For this review, take the finished solid that the model builds, in its own axes (mm). A direction names the side the tool comes from. Coordinates: 2 decimals unless noted, no trailing zeros. Loops run counter-clockwise (first coordinate to the right, second up) from the corner with the lowest first, then second, coordinate; pieces in that order, holes last. Notation, with made-up numbers: M -15.5,-3.5 L 15.5,-3.5 A19 ccw 15.5,30.5 Z; hole C -17.75,89.5 d11. An arc over 180 degrees is marked long. Put each result on its own line as item: value.
```python
from build123d import *

# Parameters (mm, degrees)
SKETCH1_R                                         = 5.08
SKETCH1_R_2                                       = 1.524
BOSS_EXTRUDE1_DEPTH                               = 1.4732
CSK_FOR_4_FLAT_HEAD_MACHINE_SCREW_100_D           = 3.4544
CSK_FOR_4_FLAT_HEAD_MACHINE_SCREW_100_DEPTH       = 3.44932
CSK_FOR_4_FLAT_HEAD_MACHINE_SCREW_100_CSINK_D     = 5.715
CSK_FOR_4_FLAT_HEAD_MACHINE_SCREW_100_CSINK_ANGLE = 100
CSK_FOR_4_FLAT_HEAD_MACHINE_SCREW_100_TIP         = 1.037806461


with BuildPart() as part:
    # Sketch1 → Boss-Extrude1 (new body)
    with BuildSketch(Plane(origin=(0, 0, 0), x_dir=(1, 0, 0), z_dir=(0, 1, 0))):
        with BuildLine():
            Line((-3.81, 7.493), (-3.81, 16.383))
            ThreePointArc((-3.81, 16.383), (-2.731274275, 18.987274275), (-0.127, 20.066))
            Line((-0.127, 20.066), (0.127, 20.066))
            ThreePointArc((0.127, 20.066), (2.731274275, 18.987274275), (3.81, 16.383))
            Line((3.81, 16.383), (3.81, 7.493))
            ThreePointArc((3.81, 7.493), (4.888725725, 4.888725725), (7.493, 3.81))
            Line((7.493, 3.81), (16.383, 3.81))
            ThreePointArc((16.383, 3.81), (18.987274275, 2.731274275), (20.066, 0.127))
            Line((20.066, 0.127), (20.066, -0.127))
            ThreePointArc((20.066, -0.127), (18.987274275, -2.731274275), (16.383, -3.81))
            Line((16.383, -3.81), (7.493, -3.81))
            ThreePointArc((7.493, -3.81), (4.888725725, -4.888725725), (3.81, -7.493))
            Line((3.81, -7.493), (3.81, -16.383))
            ThreePointArc((3.81, -16.383), (2.731274275, -18.987274275), (0.127, -20.066))
            Line((0.127, -20.066), (-0.127, -20.066))
            ThreePointArc((-0.127, -20.066), (-2.731274275, -18.987274275), (-3.81, -16.383))
            Line((-3.81, -16.383), (-3.81, -7.493))
            ThreePointArc((-3.81, -7.493), (-4.888725725, -4.888725725), (-7.493, -3.81))
            Line((-7.493, -3.81), (-16.383, -3.81))
            ThreePointArc((-16.383, -3.81), (-18.987274275, -2.731274275), (-20.066, -0.127))
            Line((-20.066, -0.127), (-20.066, 0.127))
            ThreePointArc((-20.066, 0.127), (-18.987274275, 2.731274275), (-16.383, 3.81))
            Line((-16.383, 3.81), (-7.493, 3.81))
            ThreePointArc((-7.493, 3.81), (-4.888725725, 4.888725725), (-3.81, 7.493))
        make_face()
        Circle(SKETCH1_R, mode=Mode.SUBTRACT)
        with Locations((0, 17.0815)):
            Circle(SKETCH1_R_2, mode=Mode.SUBTRACT)
        with Locations((17.0815, 0)):
            Circle(SKETCH1_R_2, mode=Mode.SUBTRACT)
        with Locations((-17.0815, 0)):
            Circle(SKETCH1_R_2, mode=Mode.SUBTRACT)
        with Locations((0, -17.0815)):
            Circle(SKETCH1_R_2, mode=Mode.SUBTRACT)
    extrude(amount=BOSS_EXTRUDE1_DEPTH)

    # CSK for #4 Flat Head Machine Screw (100)2
    with Locations(Plane(origin=(0, 1.4732, 0), x_dir=(1, 0, 0), z_dir=(0, 1, 0))):
        with Locations((0, 8.001), (0, -8.001), (9.271, 0), (-9.271, 0)):
            CounterSinkHole(CSK_FOR_4_FLAT_HEAD_MACHINE_SCREW_100_D / 2, CSK_FOR_4_FLAT_HEAD_MACHINE_SCREW_100_CSINK_D / 2, depth=CSK_FOR_4_FLAT_HEAD_MACHINE_SCREW_100_DEPTH, counter_sink_angle=CSK_FOR_4_FLAT_HEAD_MACHINE_SCREW_100_CSINK_ANGLE)
            with Locations((0, 0, -(CSK_FOR_4_FLAT_HEAD_MACHINE_SCREW_100_DEPTH + CSK_FOR_4_FLAT_HEAD_MACHINE_SCREW_100_TIP / 2))):  # 118° drill point
                Cone(0, CSK_FOR_4_FLAT_HEAD_MACHINE_SCREW_100_D / 2, CSK_FOR_4_FLAT_HEAD_MACHINE_SCREW_100_TIP, mode=Mode.SUBTRACT)


solid = part.part
```
(1) Wall thickness on line 1 along Z through (x, y) = (0, 0.15); line 2 along Z through (x, y) = (-1, 0.5); line 3 along X through (y, z) = (0.45, -8): over which ranges is each line inside the solid? List them lowest first. Write a range as [from, to].
Determined:
line 1: z = [-20.07, -18.61], [-15.56, -9.73], [-6.27, -5.08], [5.08, 6.27], [9.73, 15.56], [18.61, 20.07]
line 2: z = [-19.96, -18.23], [-15.93, -9.41], [-6.59, -4.98], [4.98, 6.59], [9.41, 15.93], [18.23, 19.96]
line 3: x = [-3.81, -1.73], [1.73, 3.81]
(2) Tool access review of faces 5 (the flat face through (2, 0, -6)), 6 (the flat face through (-3.81, 1, -12)): name each direction out of +Z, -Z, +X, -X, +Y, -Y from which nothing blocks a thin tool from reaching the whole face with its end or side.
Determined:
face 5: +Z, -Z, +X, -X, -Y
face 6: -Z, -X, +Y, -Y
(3) Draft analysis for pull direction Z (two halves, no side actions). For faces 1 (the flat face through (3.81, 1, -12)), 2 (the cylindrical face through (-0.198, 0.726, -18.593)), 3 (the cylindrical face through (19.02, 0.73, 2.7)), 4 (the cylindrical face through (0.37, 0.26, 9.69)), state which applies: +Z half, -Z half, draft (parallel to the pull), parting line (faces both ways), or undercut.
Determined:
face 1: draft
face 2: undercut
face 3: +Z half
face 4: undercut
(4) Add section C-C (z = 12). Write out the cut boundary in (x, y), plus the area to 3 significant figures.
Determined:
outline: M -3.81,0 L 3.81,0 L 3.81,1.47 L -3.81,1.47 Z
area: 11.2 mm^2
(5) Add section A-A (y = 0.25). State how many separate pieces and enclosed holes the cut face has, plus the area to 3 significant figures.
Determined:
separate pieces: 1
enclosed holes: 9
area: 394 mm^2
(6) Add section B-B (x = 17). Write out the cut boundary in (y, z).
Determined:
outline: M 0,-3.76 L 1.47,-3.76 L 1.47,-1.52 L 0,-1.52 Z; M 0,1.52 L 1.47,1.52 L 1.47,3.76 L 0,3.76 Z
(7) For pin 1 (2.5 mm diameter, centred on x = -17.08, z = 0, fed in from +Y); pin 2 (4.5 mm diameter, centred on x = 9.271, z = 0, fed in from +Y); pin 3 (0.7 mm diameter, centred on x = -13.5, y = 1, fed in from +Z), all flat-tipped, find the tip position at first contact; note any pin that passes through.
Determined:
pin 1: passes through
pin 2: stops at y = 0.96
pin 3: stops at z = 3.81
